Model file for the job. Use its own axes, mm. Face numbers are marked on the shaded views. A direction names the side the tool comes from. Give positions to 0.01 mm unless a question says otherwise; leave off trailing zeros. Order: outer loops, then holes, each group sorted by start corner. A loop starts at its lowest first (then second) coordinate and runs counter-clockwise, first axis right, second up. Notation, with made-up numbers: M 65.5,42 L 83.5,42 A31 cw 83.5,76 Z; hole C 50,84 d3. An arc over 180 degrees is marked long. Return JSON: item names as keys, results as strings. Group by question number.
1. Slice it at B-B on x = 0. List the corners of the cut face in (y, z).
2. Wall check: probe 1 along Z at (x, y) = (0.75, 3.25); probe 2 along X at (y, z) = (1.5, 3.75); probe 3 along X at (y, z) = (5.5, 5.45). Give the ranges that are in metal, low to high. Write a range as [from, to].
3. Two-plate mould, pull along X, no slides. Class the marked faces 1, 2, 3 and 4: released by +X, released by -X, zero draft, split by the parting line, or undercut.
4. Slice it at A-A on y = 4.25. List the corners of the cut face in (x, z), then the cut area to 3 significant figures.
5. Pin check, flat tip, straight feed: pin 1 (1 mm diameter, centred on x = 2.5, z = 1, fed in from +Y). Stop position of the tip, or through.
6. Slice it at C-C on z = 4.2. List the corners of the cut face in (x, y).
7. Slice it at D-D on x = 1.75. List the corners of the cut face in (y, z), then the cut area to 3 significant figures.
8. 3-axis set-ups, long thin cutter, end or side, ignore diameter. For the marked faces 5 and 6: which of +Z, -Z, +X, -X, +Y, -Y reach the whole face in a straight line?
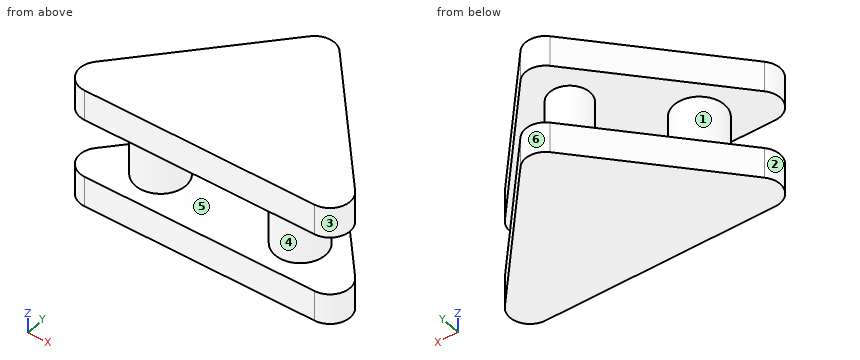
from build123d import *

# Parameters (mm, degrees)
BOSS_EXTRUDE1_DEPTH     = 6
CUT_EXTRUDE1_DEPTH      = 14.416407865
CUT_EXTRUDE1_DEPTH_BACK = 14.416407865
SKETCH2_W               = 2.938755012
SKETCH2_H               = 8.94427191
SKETCH3_R               = 1
SKETCH3_R_2             = 1.25
BOSS_EXTRUDE2_DEPTH     = 6
FILLET1_R               = 1


with BuildPart() as part:
    # Sketch1 → Boss-Extrude1 (new body)
    with BuildSketch(Plane.XY):
        Polygon((-8, 0), (8, 0), (0, 8.94427191), align=None)
    extrude(amount=BOSS_EXTRUDE1_DEPTH)

    # Sketch2 → Cut-Extrude1 (cut, two sides: drawn at the far end of the back side and taken through both)
    with BuildSketch(Plane(origin=(0, 0, 0), x_dir=(0, 0, -1), z_dir=(1, 0, 0)).offset(-CUT_EXTRUDE1_DEPTH_BACK)):
        with Locations((-3, 4.472135955)):
            Rectangle(SKETCH2_W, SKETCH2_H)
    extrude(amount=CUT_EXTRUDE1_DEPTH + CUT_EXTRUDE1_DEPTH_BACK, mode=Mode.SUBTRACT)


with BuildPart() as cut_extrude1_piece_1:
    # of the separate pieces the step leaves, piece 1, a body of its own (cut_extrude1_pieces)
    add(part.part.solids().sort_by_distance((-8, 0, 0))[0])



with BuildPart() as cut_extrude1_piece_2:
    # of the separate pieces the step leaves, piece 2, a body of its own (cut_extrude1_pieces)
    add(part.part.solids().sort_by_distance((-8, 0, 4.469377506))[0])


with BuildPart() as cut_extrude1_piece_1_1:
    add(cut_extrude1_piece_1.part)

    add(cut_extrude1_piece_2.part)  # Boss-Extrude2 merges Cut-Extrude1 piece 2
    # Sketch3 → Boss-Extrude2 (add)
    with BuildSketch(Plane.XY):
        with Locations(Location((0, 5.874639057, 0), (0, 0, 90))):
            Circle(SKETCH3_R)
        with Locations(Location((-3.5, 2, 0), (0, 0, 90))):
            Circle(SKETCH3_R_2)
        with Locations(Location((3.5, 2, 0), (0, 0, 90))):
            Circle(SKETCH3_R_2)
    extrude(amount=BOSS_EXTRUDE2_DEPTH)

    # Fillet1
    fillet1_edges = [cut_extrude1_piece_1_1.edges().sort_by_distance(p)[0] for p in [
        (-8, 0, 5.234688753),
        (8, 0, 0.765311247),
        (-8, 0, 0.765311247),
        (0, 8.94427191, 0.765311247),
        (8, 0, 5.234688753),
        (0, 8.94427191, 5.234688753),
    ]]
    fillet(fillet1_edges, radius=FILLET1_R)


solid = cut_extrude1_piece_1_1.part
Result:
{
 "1": {"outline": "M 0,0 L 8.44,0 L 8.44,1.53 L 6.87,1.53 L 6.87,4.47 L 8.44,4.47 L 8.44,6 L 0,6 L 0,4.47 L 4.87,4.47 L 4.87,1.53 L 0,1.53 Z"},
 "2": {"probe 1": "z = [0, 1.53], [4.47, 6]", "probe 2": "x = [-4.65, -2.35], [2.35, 4.65]", "probe 3": "x = [-3.08, 3.08]"},
 "3": {"face 1": "undercut", "face 2": "released by -X", "face 3": "released by +X", "face 4": "undercut"},
 "4": {"outline": "M -4.2,0 L 4.2,0 L 4.2,1.53 L -4.2,1.53 Z; M -4.2,4.47 L 4.2,4.47 L 4.2,6 L -4.2,6 Z", "area": "25.7 mm2"},
 "5": {"pin 1": "stops at y = 6.71"},
 "6": {"outline": "C -3.5,2 d2.5; C 0,5.87 d2; C 3.5,2 d2.5"},
 "7": {"outline": "M 0,0 L 6.99,0 L 6.99,1.53 L 0,1.53 Z; M 0,4.47 L 6.99,4.47 L 6.99,6 L 0,6 Z", "area": "21.4 mm2"},
 "8": {"face 5": "none", "face 6": "+Z, -Z, +Y"}
}
